The listing builds one solid part. Answer for the finished solid, in the listing's coordinates (mm). Face numbers are marked on the shaded views. Coordinates: 2 decimals unless noted, no trailing zeros. Write each loop counter-clockwise with the first axis right and the second up, starting at its lowest first coordinate (ties: lowest second). Pieces come first, ordered by that corner, then holes.
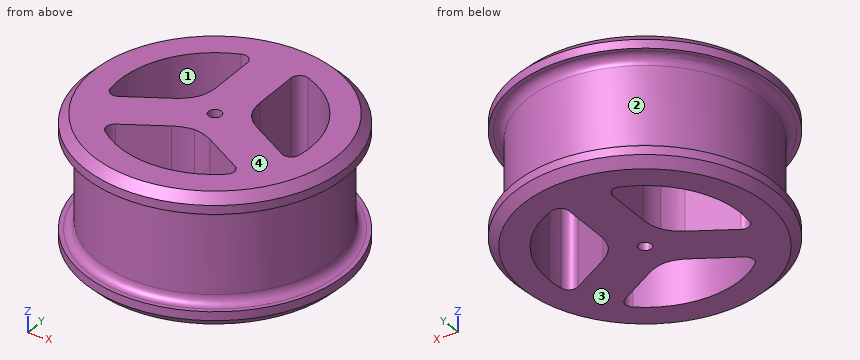
from build123d import *

# Parameters (mm, degrees)
SKETCH1_R           = 15
SKETCH1_R_2         = 0.75
BOSS_EXTRUDE1_DEPTH = 15
CUT_EXTRUDE1_START  = -11
SKETCH2_R           = 15
SKETCH2_R_2         = 13.5
CUT_EXTRUDE1_DEPTH  = 11
FILLET1_R           = 1
CUT_EXTRUDE2_DEPTH  = 26.980762114
FILLET2_R           = 5
FILLET3_R           = 1
CHAMFER2_SIZE       = 1


with BuildPart() as part:
    # Sketch1 → Boss-Extrude1 (new body)
    with BuildSketch(Plane.XY):
        Circle(SKETCH1_R)
        Circle(SKETCH1_R_2, mode=Mode.SUBTRACT)
    extrude(amount=BOSS_EXTRUDE1_DEPTH)

    # Sketch2 → Cut-Extrude1 (cut)
    with BuildSketch(Plane.XY.offset(13).offset(CUT_EXTRUDE1_START)):
        Circle(SKETCH2_R)
        Circle(SKETCH2_R_2, mode=Mode.SUBTRACT)
    extrude(amount=CUT_EXTRUDE1_DEPTH, mode=Mode.SUBTRACT)

    # Fillet1
    fillet1_edges = [part.edges().sort_by_distance(p)[0] for p in [
        (-13.5, 0, 2),
        (-13.5, 0, 13),
    ]]
    fillet(fillet1_edges, radius=FILLET1_R)

    # Sketch4 → Cut-Extrude2 (cut, through all)
    with BuildSketch(Plane.XY.offset(15)):
        with BuildLine():
            Line((2.5, 10.712142643), (2.5, 2.449489743))
            ThreePointArc((2.5, 2.449489743), (3.031088913, 1.75), (3.371320344, 0.940318638))
            Line((3.371320344, 0.940318638), (10.526987658, -3.191007812))
            ThreePointArc((10.526987658, -3.191007812), (10.881104361, -1.612937656), (11, 0))
            ThreePointArc((11, 0), (8.61684397, 6.837397166), (2.5, 10.712142643))
        make_face()
        with BuildLine():
            ThreePointArc((-8.026987658, -7.521134831), (0, -11), (8.026987658, -7.521134831))
            Line((8.026987658, -7.521134831), (0.871320344, -3.389808381))
            ThreePointArc((0.871320344, -3.389808381), (0, -3.5), (-0.871320344, -3.389808381))
            Line((-0.871320344, -3.389808381), (-8.026987658, -7.521134831))
        make_face()
        with BuildLine():
            ThreePointArc((-3.371320344, 0.940318638), (-3.031088913, 1.75), (-2.5, 2.449489743))
            Line((-2.5, 2.449489743), (-2.5, 10.712142643))
            ThreePointArc((-2.5, 10.712142643), (-9.526279442, 5.5), (-10.526987658, -3.191007812))
            Line((-10.526987658, -3.191007812), (-3.371320344, 0.940318638))
        make_face()
    extrude(amount=-CUT_EXTRUDE2_DEPTH, mode=Mode.SUBTRACT)

    # Fillet2
    # the kernel refuses this fillet: 5 mm, written as the material it adds along each edge
    with BuildSketch(Plane(origin=(-0.871320344, -3.389808381, 15), x_dir=(0.994067927349263, -0.108761003192966, 0), z_dir=(0, 0, -1)), Plane(origin=(3.371320344, 0.940318638, 15), x_dir=(-0.40284417196844124, 0.9152685797682891, 0), z_dir=(0, 0, -1)), Plane(origin=(-2.5, 2.449489743, 15), x_dir=(-0.5912237553808212, -0.8065075765753221, 0), z_dir=(0, 0, -1))) as fillet2_piece_1:
        with BuildLine():
            CenterArc((1.705620507, 4.94923638), FILLET2_R, 233.756102233, 28.072486936)
            Line((-1.25049827, 0.916698497), (0, 0))
            ThreePointArc((0, 0), (0.497472648, 0.035534534), (0.994945296, 0))
        make_face()
    extrude(amount=15)
    with BuildSketch(Plane(origin=(0.871320344, -3.389808381, 15), x_dir=(0.8660254037844362, -0.5000000000000042, 0), z_dir=(0, 0, -1)), Plane(origin=(2.5, 2.449489743, 15), x_dir=(0, 1, 0), z_dir=(0, 0, -1)), Plane(origin=(-3.371320344, 0.940318638, 15), x_dir=(-0.8660254037844451, -0.49999999999998884, 0), z_dir=(0, 0, -1))) as fillet2_piece_2:
        with BuildLine():
            CenterArc((1.550510257, 5), FILLET2_R, 241.927513064, 28.072486936)
            ThreePointArc((-0.802430919, 0.588235294), (-0.380206599, 0.322776518), (0, 0))
            Line((0, 0), (1.550510257, 0))
        make_face()
    extrude(amount=15)

    # Fillet3
    fillet3_edges = [part.edges().sort_by_distance(p)[0] for p in [
        (-2.5, 10.712142643, 7.5),
        (-10.526987658, -3.191007812, 7.5),
        (-8.026987658, -7.521134831, 7.5),
        (8.026987658, -7.521134831, 7.5),
        (10.526987658, -3.191007812, 7.5),
        (2.5, 10.712142643, 7.5),
    ]]
    fillet(fillet3_edges, radius=FILLET3_R)

    # Chamfer2
    chamfer2_edges = [part.edges().sort_by_distance(p)[0] for p in [
        (-15, 0, 0),
        (-15, 0, 15),
    ]]
    chamfer(chamfer2_edges, length=CHAMFER2_SIZE)


solid = part.part
Q1. The part is cut by section B-B, the plane z = 13.5. Write down the section's boundary in (x, y).
Answers below:
outline: circle Ø30 at (0, 0); hole (-10.85, -1.82) arc R1 ccw to (-9.36, -2.52) - (-4.71, 0.17) arc R5 ccw to (-3.03, 1.75) arc R5 ccw to (-2.5, 4) - (-2.5, 9.37) arc R1 ccw to (-3.85, 10.3) arc R11 ccw to start; hole (-7, -8.49) arc R11 ccw to (7, -8.49) arc R1 ccw to (6.86, -6.85) - (2.21, -4.17) arc R5 ccw to (0, -3.5) arc R5 ccw to (-2.21, -4.17) - (-6.86, -6.85) arc R1 ccw to start; hole circle Ø1.5 at (0, 0); hole (2.5, 4) arc R5 ccw to (3.03, 1.75) arc R5 ccw to (4.71, 0.17) - (9.36, -2.52) arc R1 ccw to (10.85, -1.82) arc R11 ccw to (3.85, 10.3) arc R1 ccw to (2.5, 9.37) - close
Q2. The part is cut by section A-A, the plane z = 11.25. Write down the section's boundary in (x, y).
Answers below:
outline: circle Ø27 at (0, 0); hole (-10.85, -1.82) arc R1 ccw to (-9.36, -2.52) - (-4.71, 0.17) arc R5 ccw to (-3.03, 1.75) arc R5 ccw to (-2.5, 4) - (-2.5, 9.37) arc R1 ccw to (-3.85, 10.3) arc R11 ccw to start; hole (-7, -8.49) arc R11 ccw to (7, -8.49) arc R1 ccw to (6.86, -6.85) - (2.21, -4.17) arc R5 ccw to (0, -3.5) arc R5 ccw to (-2.21, -4.17) - (-6.86, -6.85) arc R1 ccw to start; hole circle Ø1.5 at (0, 0); hole (2.5, 4) arc R5 ccw to (3.03, 1.75) arc R5 ccw to (4.71, 0.17) - (9.36, -2.52) arc R1 ccw to (10.85, -1.82) arc R11 ccw to (3.85, 10.3) arc R1 ccw to (2.5, 9.37) - close
Q3. Given pin 1 (2.5 mm diameter, centred on y = 6.5, z = 8, fed in from -X); pin 2 (3 mm diameter, centred on y = -6, z = 8.5, fed in from -X); pin 3 (0.9 mm diameter, centred on x = 0, y = 0, fed in from -Z); pin 4 (6 mm diameter, centred on x = -5.5, z = 5.5, fed in from -Y), each flat-ended and moving along its own axis, determine where each tip first touches the part or whether it passes through.
Answers below:
pin 1: stops at x = -12.44
pin 2: stops at x = -12.73
pin 3: passes through
pin 4: stops at y = -13.27
Q4. Find the intervals of material crossed by probe 1 along Y at (x, z) = (-5.5, 8.75); probe 2 along X at (y, z) = (-4.5, 9.75); probe 3 along X at (y, z) = (-1.25, 11.75), in increasing order.
Answers below:
probe 1: y = -12.33 to -9.53, -6.06 to -0.29, 9.53 to 12.33
probe 2: x = -12.73 to -2.79, 2.79 to 12.73
probe 3: x = -13.44 to -10.93, -7.17 to 7.17, 10.93 to 13.44
Q5. Determine the mould class of the marked faces 1, 2, 3 and 4 for opening direction Z: released by +Z, released by -Z, zero draft, split by the parting line, or undercut.
Answers below:
face 1: zero draft
face 2: undercut
face 3: released by -Z
face 4: released by +Z
Q6. The part is cut by section C-C, the plane y = 7.75. State how many separate pieces and enclosed holes the cut face has, then the cut area to 3 significant figures.
Answers below:
separate pieces: 3
enclosed holes: 0
area: 185 mm2
